Design review of the part built by this model. Coordinates are the model's own, in mm. A direction names the side the tool comes from. Give positions to 0.01 mm unless a question says otherwise; leave off trailing zeros. Order: outer loops, then holes, each group sorted by start corner. A loop starts at its lowest first (then second) coordinate and runs counter-clockwise, first axis right, second up. Notation, with made-up numbers: M 11,-22 L 67,-22 A37 cw 67,15 Z; hole C 59.5,60 d9. An arc over 180 degrees is marked long. Answer as a JSON object with one key per item and string values.
Autodesk Inventor part; units mm, degrees
ref_plane "YZ Plane" through (0, 0, 0) normal (1, 0, 0) x (0, 1, 0)
ref_plane "XZ Plane" through (0, 0, 0) normal (0, 1, 0) x (-1, 0, 0)
ref_plane "XY Plane" through (0, 0, 0) normal (0, 0, 1) x (1, 0, 0)
sketch "Sketch1" plane through (0, 0, 0) normal (0, 0, 1) x (1, 0, 0)
  line L0 (4.5, -3.75) -> (-4.5, -3.75)
  line L1 (-4.5, -3.75) -> (-4.5, 3.75)
  line L2 (-4.5, 3.75) -> (4.5, 3.75)
  line L3 (4.5, 3.75) -> (4.5, -3.75)
  line L4 (4.5, -3.75) -> (-4.5, 3.75) construction
  line L5 (-4.5, -3.75) -> (4.5, 3.75) construction
  point P0 (0, 0)
  dimension "d0" = 9
  dimension "d1" = 7.5
extrude "Extrusion1" add sketch "Sketch1" along normal mid plane 2
sketch "Sketch2" plane through (4.5, -3.75, 1) normal (1, 0, 0) x (0, 0, -1)
  line L0 (2, 7.5) -> (0, 7.5)
  line L1 (2, 7.5) -> (0, 7.5)
  line L2 (0, 7.5) -> (0, 5.5)
  line L3 (0, 5.5) -> (2, 5.5)
  line L4 (2, 5.5) -> (2, 7.5)
  point P0 (1, 3.75)
  dimension "d4" = 2
  dimension "d5" = 2
extrude "Extrusion2" add sketch "Sketch2" along normal blind 2
sketch "Sketch3" plane through (-4.5, -3.75, 1) normal (-1, 0, 0) x (0, 0, 1)
  line L0 (-2, 7.5) -> (0, 7.5)
  line L1 (0, 7.5) -> (0, 0)
  line L2 (-2, 7.5) -> (0, 7.5)
  line L3 (0, 7.5) -> (0, 5.5)
  line L4 (0, 5.5) -> (-2, 5.5)
  line L5 (-2, 5.5) -> (-2, 7.5)
  point P0 (-1, 3.75)
  dimension "d8" = 2
extrude "Extrusion3" add sketch "Sketch3" along normal blind 2
fillet "Fillet1" radius 0.1 2 edges at (4.5, 1.75, 0) (-4.5, 1.75, 0)
properties part number "Tapa_1_TFM"
(1) Draft analysis for pull direction Y (two halves, no side actions). For faces 1 (the flat face through (0, -3.75, 0)), 2 (the flat face through (6.5, 3, 0)), 3 (the flat face through (0, 3.75, 0)), state which applies: +Y half, -Y half, draft (parallel to the pull), parting line (faces both ways), or undercut.
Checked values:
{"face 1": "-Y half", "face 2": "draft", "face 3": "+Y half"}
(2) To check wall thickness, follow L1, parallel to X at y = 1.5, z = 0.85; L2, parallel to Y at x = -5.25, z = 0.2. State the ranges of each line that lie inside material, in increasing order. Write a range as from..to.
Checked values:
{"L1": "x = -4.5..4.5", "L2": "y = 1.75..3.75"}
(3) Tool access review of faces 4 (the flat face through (0, 0, 1)), 5 (the flat face through (-6, 1.75, 0)), 6 (the flat face through (4.5, -1, 0)): name each direction out of +Z, -Z, +X, -X, +Y, -Y from which nothing blocks a thin tool from reaching the whole face with its end or side.
Checked values:
{"face 4": "+Z, +X, -X, +Y, -Y", "face 5": "+Z, -Z, -X, -Y", "face 6": "+Z, -Z, +X, -Y"}
(4) We need section C-C (x = 5.75). Write out the cut boundary in (y, z), plus the area to 3 significant figures.
Checked values:
{"outline": "M 1.75,-1 L 3.75,-1 L 3.75,1 L 1.75,1 Z", "area": "4.00 mm^2"}
(5) Insertion check: pin 1 (1 mm diameter, centred on x = 5.5, z = 0.5, fed in from -Y). The pin has a flat end and moves straight along its axis. Give the tip position at first contact, or say it passes through.
Checked values:
{"pin 1": "stops at y = 1.75"}
(6) We need section A-A (z = -0.3). Write out the cut boundary in (x, y).
Checked values:
{"outline": "M -6.5,1.75 L -4.6,1.75 A0.1 cw -4.5,1.65 L -4.5,-3.75 L 4.5,-3.75 L 4.5,1.65 A0.1 cw 4.6,1.75 L 6.5,1.75 L 6.5,3.75 L -6.5,3.75 Z"}
(7) We need section B-B (y = -2). Write out the cut boundary in (x, z).
Checked values:
{"outline": "M -4.5,-1 L 4.5,-1 L 4.5,1 L -4.5,1 Z"}
